Here's how the part is built. I have some questions about the finished solid (model axes, mm). Round coordinates to 2 decimals unless told otherwise and drop trailing zeros. Loops run counter-clockwise (first coordinate to the right, second up) from the corner with the lowest first, then second, coordinate; pieces in that order, holes last. Notation, with made-up numbers: M 53.5,-23.5 L 100.5,-23.5 A11 cw 100.5,-14.5 Z; hole C 35.25,-30.5 d7. An arc over 180 degrees is marked long. Answer as CSV lines item,"result".
```python
from build123d import *

# Parameters (mm, degrees)
SKETCH1_R           = 3.5
BOSS_EXTRUDE1_DEPTH = 3


with BuildPart() as part:
    # Sketch1 → Boss-Extrude1 (new body)
    with BuildSketch(Plane(origin=(0, 0, 0), x_dir=(1, 0, 0), z_dir=(0, 1, 0))):
        with BuildLine():
            Line((-8.711687898, 0.175603251), (-8.711687898, 33.175603251))
            ThreePointArc((-8.711687898, 33.175603251), (-1.211687898, 40.675603251), (6.288312102, 33.175603251))
            Line((6.288312102, 33.175603251), (6.288312102, 0.175603251))
            Line((6.288312102, 0.175603251), (-8.711687898, 0.175603251))
        make_face()
        with Locations((-1.211687898, 33.175603251)):
            Circle(SKETCH1_R, mode=Mode.SUBTRACT)
    extrude(amount=BOSS_EXTRUDE1_DEPTH)


solid = part.part
```
1. We'd pull the mould along X, two halves only. Please class faces 1 (the cylindrical face through (-1.97, 1.48, -29.76)), 2 (the flat face through (6.288, 1, -17)), 3 (the flat face through (-1, 1, -0.176)), 4 (the cylindrical face through (-1.377, 1.479, -40.674)): pulls with the +X half, pulls with the -X half, needs draft (parallel to the pull), parting line crosses it, or undercut.
Evaluation:
face 1,"undercut"
face 2,"pulls with the +X half"
face 3,"needs draft"
face 4,"parting line crosses it"
2. If I drill on line 1 (Z direction, x = -2.25, y = 0.9); line 2 (Z direction, x = -1.5, y = 0.6); line 3 (X direction, y = 2, z = -35.5), over which ranges is the centre line in solid material (lowest first)? Write a range as [from, to].
Evaluation:
line 1,"z = [-40.6, -36.52], [-29.83, -0.18]"
line 2,"z = [-40.67, -36.66], [-29.69, -0.18]"
line 3,"x = [-8.34, -3.83], [1.41, 5.92]"
3. I want a section at A-A, the plane y = 2.45. Please give me the cut outline in (x, z).
Evaluation:
outline,"M -8.71,-33.18 A7.5 ccw 6.29,-33.18 L 6.29,-0.18 L -8.71,-0.18 Z; hole C -1.21,-33.18 d7"
4. I want a section at C-C, the plane z = -32.5. Please give me the cut outline in (x, y).
Evaluation:
outline,"M -8.71,0 L -4.65,0 L -4.65,3 L -8.71,3 Z; M 2.22,0 L 6.29,0 L 6.29,3 L 2.22,3 Z"
5. For P1, Ø6.5, axis at x = -1.21, z = -33.18, coming from the +Y side; P2, Ø1.5, axis at x = 1.5, y = 0.5, coming from the -Z side, each with a flat end and sliding along its axis, tell me the tip position at first contact or that it passes through.
Evaluation:
P1,"passes through"
P2,"stops at z = -40.41"
6. I want a section at B-B, the plane x = 1.5. Please give me the cut outline in (y, z).
Evaluation:
outline,"M 0,-40.17 L 3,-40.17 L 3,-35.39 L 0,-35.39 Z; M 0,-30.96 L 3,-30.96 L 3,-0.18 L 0,-0.18 Z"
7. I want a section at D-D, the plane x = -5.5. Please give me the cut outline in (y, z).
Evaluation:
outline,"M 0,-39.33 L 3,-39.33 L 3,-0.18 L 0,-0.18 Z"
